Here's how the part is built. I have some questions about the finished solid (model axes, mm). A direction names the side the tool comes from. Round coordinates to 2 decimals unless told otherwise and drop trailing zeros. Loops run counter-clockwise (first coordinate to the right, second up) from the corner with the lowest first, then second, coordinate; pieces in that order, holes last. Notation, with made-up numbers: M -18,89 L 6,89 A23 ccw 6,116 Z; hole C -21,-1 d1. An arc over 180 degrees is marked long. Write item = value, one per line. Start each with the question number.
from build123d import *

# Parameters (mm, degrees)
SKETCH1_R                 = 76.2
BOSS_EXTRUDE1_DEPTH       = 6.35
TAP_DRILL_FOR_6_32_TAP1_D = 2.7051
CIRPATTERN1_COUNT         = 4
W_0_386_DIAMETER_HOLE1_D  = 9.8044
CUT_EXTRUDE4_DEPTH        = 3.175
SKETCH15_R                = 76.2
SKETCH15_R_2              = 74.041
CUT_EXTRUDE5_DEPTH        = 3.175
BODY_MOVE_COPY1_ANGLE     = 40


with BuildPart() as part:
    # Sketch1 → Boss-Extrude1 (new body)
    with BuildSketch(Plane(origin=(0, 0, 0), x_dir=(1, 0, 0), z_dir=(0, 1, 0))):
        Circle(SKETCH1_R)
    extrude(amount=BOSS_EXTRUDE1_DEPTH)

    # Tap Drill for #6-32 Tap1 (through all)
    with Locations(Plane(origin=(0, 0, 0), x_dir=(-1, 0, 0), z_dir=(0, -1, 0))):
        with Locations((37.52117539, 6.615995569)):
            tap_drill_for_6_32_tap1 = Hole(TAP_DRILL_FOR_6_32_TAP1_D / 2)

    # CirPattern1: Tap Drill for #6-32 Tap1 ×4 about axis
    cirpattern1_axis = Axis((0, 0, 0), (0, 1, 0))
    for i in range(1, CIRPATTERN1_COUNT):
        add(tap_drill_for_6_32_tap1.rotate(cirpattern1_axis, i * 360 / CIRPATTERN1_COUNT), mode=Mode.SUBTRACT)

    # W (0.386) Diameter Hole1 (through all)
    with Locations(Plane(origin=(0, 0, 0), x_dir=(-1, 0, 0), z_dir=(0, -1, 0))):
        with Locations((-33.077799054, 27.755568986), (33.077799054, -27.755568986)):
            Hole(W_0_386_DIAMETER_HOLE1_D / 2)

    # Sketch11 → 3/16 (0.1875) Diameter Hole1 (revolve, cut)
    with BuildSketch(Plane(origin=(-18.760587695, 0, -3.307997785), x_dir=(0, 0, -1), z_dir=(1, 0, 0))):
        Polygon((0, 0), (0, 6.35), (3.01625, 6.35), (2.38125, 5.715), (2.38125, 0.635), (3.01625, 0), align=None)
    revolve(axis=Axis((-18.760587695, -6.35, -3.307997785), (0, 1, 0)), mode=Mode.SUBTRACT)

    # Sketch12 → Cut-Extrude4 (cut)
    with BuildSketch(Plane.XZ):
        with BuildLine():
            ThreePointArc((24.848558171, 24.575146858), (20.286055568, 24.175979603), (19.886888313, 28.738482206))
            Line((19.886888313, 28.738482206), (6.498907978, 12.783308544))
            ThreePointArc((6.498907978, 12.783308544), (10.087375141, 13.744835423), (12.218242907, 10.70164087))
            ThreePointArc((12.218242907, 10.70164087), (12.02293746, 9.594008636), (11.460577836, 8.619973196))
            Line((11.460577836, 8.619973196), (24.848558171, 24.575146858))
        make_face()
        with BuildLine():
            ThreePointArc((25.606223242, 26.656814532), (23.475355476, 29.700009084), (19.886888313, 28.738482206))
            Line((19.886888313, 28.738482206), (24.848558171, 24.575146858))
            ThreePointArc((24.848558171, 24.575146858), (25.410917794, 25.549182297), (25.606223242, 26.656814532))
        make_face()
        with BuildLine():
            Line((24.848558171, 24.575146858), (19.886888313, 28.738482206))
            ThreePointArc((19.886888313, 28.738482206), (20.286055568, 24.175979603), (24.848558171, 24.575146858))
        make_face()
        with BuildLine():
            ThreePointArc((12.218242907, 10.70164087), (10.087375141, 13.744835423), (6.498907978, 12.783308544))
            Line((6.498907978, 12.783308544), (11.460577836, 8.619973196))
            ThreePointArc((11.460577836, 8.619973196), (12.02293746, 9.594008636), (12.218242907, 10.70164087))
        make_face()
        with BuildLine():
            Line((11.460577836, 8.619973196), (6.498907978, 12.783308544))
            ThreePointArc((6.498907978, 12.783308544), (6.898075233, 8.220805941), (11.460577836, 8.619973196))
        make_face()
    cut_extrude4 = extrude(amount=-CUT_EXTRUDE4_DEPTH, mode=Mode.SUBTRACT)

    # Mirror1: Cut-Extrude4 across plane
    add(cut_extrude4.mirror(Plane(origin=(0, 0, 0), x_dir=(-0.766044443, 0, 0.64278761), z_dir=(0.64278761, 0, 0.766044443))), mode=Mode.SUBTRACT)

    # Sketch15 → Cut-Extrude5 (cut)
    with BuildSketch(Plane.XZ):
        Circle(SKETCH15_R)
        Circle(SKETCH15_R_2, mode=Mode.SUBTRACT)
    extrude(amount=-CUT_EXTRUDE5_DEPTH, mode=Mode.SUBTRACT)


with BuildPart() as part_1:
    # Body-Move/Copy1: moved
    add(part.part.rotate(Axis((0, 0, 0), (0, -1, 0)), BODY_MOVE_COPY1_ANGLE))


solid = part_1.part
Item 1: Please list where these lines run through material, in increasing order: line 1 (X direction, y = 4.5, z = 0); line 2 (Z direction, x = -2.5, y = 1.75); line 3 (X direction, y = 4, z = 25.5). Write a range as [from, to].
Item 2: Will these pins go through, and if not, where does the flat tip stop? pin 1 Ø1 at (y, z) = (3, -30.5) entering from +X; pin 2 Ø8 at (x, z) = (43.18, 0) entering from -Y; pin 3 Ø3.5 at (y, z) = (1, -23.5) entering from -X; pin 4 Ø1 at (y, z) = (2, 11) entering from -X.
Item 3: We'd pull the mould along Z, two halves only. Please class faces 3 (the cylindrical face through (-73.97, 1.57, 3.26)), 4 (the cylindrical face through (-10.13, 3.14, -15.69)), 5 (the flat face through (0, 6.35, -2)), 6 (the flat face through (0, 3.175, -24)): released by +Z, released by -Z, zero draft, split by the parting line, or undercut.
Item 4: For faces 1 (the cylindrical face through (70.389, 4.74, 29.185)), 2 (the flat face through (-71, 3.175, 22)), which set-ups out of +Z, -Z, +X, -X, +Y, -Y let a thin tool reach every point of the face, with its end or its side?
Item 5: I want a section at B-B, the plane x = -43.18. List the corners of the cut face in (y, z) for me (3 decimals).
Item 6: I want a section at C-C, the plane y = 1.75. State how many separate pieces and enclosed holes the cut face has, then the cut area to 3 significant figures.
Item 7: I want a section at A-A, the plane z = 0. List the corners of the cut face in (x, y) for me (3 decimals), then the cut area to 3 significant figures.
Worked out:
q1.line_1 = [-76.2, -48.08], [-38.28, 38.28], [48.08, 76.2]
q1.line_2 = [-74, -36.86], [-11.91, 11.91], [36.86, 74]
q1.line_3 = [-71.81, -30.09], [-28.29, 71.81]
q2.pin_1 = 70.03
q2.pin_2 = through
q2.pin_3 = -70.77
q2.pin_4 = -73.29
q3.face_3 = split by the parting line
q3.face_4 = undercut
q3.face_5 = zero draft
q3.face_6 = undercut
q4.face_1 = +Y, -Y
q4.face_2 = -Y
q5.outline = M 0,-60.146 L 3.175,-60.146 L 3.175,-62.785 L 6.35,-62.785 L 6.35,-4.902 L 0,-4.902 Z; M 0,4.902 L 6.35,4.902 L 6.35,62.785 L 3.175,62.785 L 3.175,60.146 L 0,60.146 Z
q6.separate_pieces = 1
q6.enclosed_holes = 9
q6.area = 16,700 mm2
q7.outline = M -76.2,3.175 L -74.041,3.175 L -74.041,0 L -48.082,0 L -48.082,6.35 L -76.2,6.35 Z; M -38.278,0 L 38.278,0 L 38.278,6.35 L -38.278,6.35 Z; M 48.082,0 L 74.041,0 L 74.041,3.175 L 76.2,3.175 L 76.2,6.35 L 48.082,6.35 Z
q7.area = 830 mm2
